Verification items for the finished model (mm, model axes). A direction names the side the tool comes from. Give positions to 0.01 mm unless a question says otherwise; leave off trailing zeros. Write each loop counter-clockwise with the first axis right and the second up, starting at its lowest first coordinate (ties: lowest second). Pieces come first, ordered by that corner, then holes.
from build123d import *

# Parameters (mm, degrees)
F0_R     = 1.55
F1_DEPTH = 2.5
F3_DEPTH = 2.501
F4_W     = 6.5
F4_H     = 1
F5_DEPTH = 1
F6_W     = 6.5
F6_H     = 1
F7_DEPTH = 1
F8_SIZE  = 0.99999


# Not quite as in the source:
# - a fillet or chamfer is up to 0.001 mm smaller than in the source, because OpenCascade refuses the exact size


with BuildPart() as f1:
    # F0 (on Top) → F1 (new body)
    with BuildSketch(Plane.XY):
        with BuildLine():
            Line((7, 4), (-7, 4))
            ThreePointArc((-7, 4), (-9.8284271247, 2.8284271247), (-11, 0))
            ThreePointArc((-11, 0), (-9.8284271247, -2.8284271247), (-7, -4))
            Line((-7, -4), (7, -4))
            ThreePointArc((7, -4), (9.8284271247, -2.8284271247), (11, 0))
            ThreePointArc((11, 0), (9.8284271247, 2.8284271247), (7, 4))
        make_face()
        with Locations((-7, 0)):
            Circle(F0_R, mode=Mode.SUBTRACT)
        with Locations((7, 0)):
            Circle(F0_R, mode=Mode.SUBTRACT)
    extrude(amount=F1_DEPTH)

    # F2 (on face) → F3 (cut, through all)
    with BuildSketch(Plane.XY.offset(2.5)):
        with BuildLine():
            Line((-7, 1.55), (-7, 4))
            ThreePointArc((-7, 4), (-11, 0), (-7, -4))
            Line((-7, -4), (-7, -1.55))
            ThreePointArc((-7, -1.55), (-8.55, 0), (-7, 1.55))
        make_face()
        with BuildLine():
            ThreePointArc((7, -4), (11, 0), (7, 4))
            Line((7, 4), (7, 1.55))
            ThreePointArc((7, 1.55), (8.0960155108, 1.0960155108), (8.55, 0))
            ThreePointArc((8.55, 0), (8.0960155108, -1.0960155108), (7, -1.55))
            Line((7, -1.55), (7, -4))
        make_face()
    extrude(amount=-F3_DEPTH, mode=Mode.SUBTRACT)

    # F4 (on face) → F5 (cut)
    with BuildSketch(Plane.XY.offset(2.5)):
        with Locations((0, 1.5)):
            Rectangle(F4_W, F4_H)
        with Locations((0, -2.5)):
            Rectangle(F4_W, F4_H)
        with Locations((0, -0.5)):
            Rectangle(F4_W, F4_H)
        with Locations((0, 3.5)):
            Rectangle(F4_W, F4_H)
    extrude(amount=-F5_DEPTH, mode=Mode.SUBTRACT)

    # F6 (on face) → F7 (cut)
    with BuildSketch(Plane(origin=(0, 0, 0), x_dir=(1, 0, 0), z_dir=(0, 0, -1))):
        with Locations((0, -0.5)):
            Rectangle(F6_W, F6_H)
        with Locations((0, 3.5)):
            Rectangle(F6_W, F6_H)
        with Locations((0, 1.5)):
            Rectangle(F6_W, F6_H)
        with Locations((0, -2.5)):
            Rectangle(F6_W, F6_H)
    extrude(amount=-F7_DEPTH, mode=Mode.SUBTRACT)

    # F8 (size 1 in the source; OpenCascade refuses exactly that, so slightly less here)
    f8_edges = [f1.edges().sort_by_distance(p)[0] for p in [
        (0, 3, 0),
        (0, 1, 0),
        (0, -1, 0),
        (0, -3, 0),
        (0, -4, 2.5),
        (0, -2, 2.5),
        (0, 0, 2.5),
        (0, 2, 2.5),
    ]]
    chamfer(f8_edges, length=F8_SIZE)


solid = f1.part
Item 1: Sectioned sample at B-B on z = 1.2. Record the cut outline in (x, y), then the cut area to 3 significant figures.
Answer key:
outline: (-7, -4) - (7, -4) - (7, -1.55) arc R1.55 cw to (7, 1.55) - (7, 4) - (-7, 4) - (-7, 1.55) arc R1.55 cw to (-7, -1.55) - close
area: 104 mm2
Item 2: Depth check by flat-ended pin: pin 1 (1.1 mm diameter, centred on x = -0.5, z = 2, fed in from +Y); pin 2 (1.1 mm diameter, centred on y = 0, z = 2, fed in from +X). Enter the tip coordinate at first touch or a pass-through.
Answer key:
pin 1: stops at y = 4
pin 2: stops at x = 5.55
Item 3: Sectioned sample at A-A on y = 2.5. Record the cut outline in (x, z), then the cut area to 4 significant figures.
Answer key:
outline: (-7, 0) - (-3.25, 0) - (-3.25, 1) - (3.25, 1) - (3.25, 0) - (7, 0) - (7, 2.5) - (3.25, 2.5) - (3.25, 2) - (-3.25, 2) - (-3.25, 2.5) - (-7, 2.5) - close
area: 25.25 mm2
Item 4: Release check for a two-part mould opening along Y. For faces 1 (the face through (-0.1, -4, 1.2)), 2 (the face through (-7, -3, 1)), 3 (the face through (0, -0.5, 1.5)) record: released by +Y, released by -Y, zero draft, split by the parting line, or undercut.
Answer key:
face 1: released by -Y
face 2: zero draft
face 3: undercut
Item 5: Sectioned sample at D-D on y = -2.75. Record the cut outline in (x, z).
Answer key:
outline: (-7, 0) - (-3.25, 0) - (-3.25, 0.75) - (3.25, 0.75) - (3.25, 0) - (7, 0) - (7, 2.5) - (3.25, 2.5) - (3.25, 1.5) - (-3.25, 1.5) - (-3.25, 2.5) - (-7, 2.5) - close
Item 6: Scan lines: line 1 along Y through (x, z) = (-1.25, 1.9); line 2 along X through (y, z) = (-2, 1.6); line 3 along Y through (x, z) = (-1, 1.65). Record each from-to range of solid material in increasing order.
Answer key:
line 1: y = -3.6 to -3, -1.6 to -1, 0.4 to 1, 2.4 to 3
line 2: x = -7 to -3.25, 3.25 to 7
line 3: y = -3.85 to -3, -1.85 to -1, 0.15 to 1, 2.15 to 3
Item 7: Sectioned sample at C-C on z = 2.15. Record the cut outline in (x, y).
Answer key:
outline: (-7, -3.35) - (7, -3.35) - (7, -1.55) arc R1.55 cw to (7, 1.55) - (7, 4) - (3.25, 4) - (3.25, 3) - (-3.25, 3) - (-3.25, 4) - (-7, 4) - (-7, 1.55) arc R1.55 cw to (-7, -1.55) - close; hole (-3.25, -3) - (3.25, -3) - (3.25, -1.35) - (-3.25, -1.35) - close; hole (-3.25, -1) - (3.25, -1) - (3.25, 0.65) - (-3.25, 0.65) - close; hole (-3.25, 1) - (3.25, 1) - (3.25, 2.65) - (-3.25, 2.65) - close
Item 8: Set-up check for faces 4 (the face through (0, -1.5, 1)), 5 (the face through (-3.25, -3.2, 0.5)), 6 (the face through (0, 2.5, 2)), 7 (the face through (7, 3, 1)), 8 (the face through (5.45, 0.03, 1.23)): record each of +Z, -Z, +X, -X, +Y, -Y from which the full face is reachable in a straight line by a thin tool's end or side.
Answer key:
face 4: -Z
face 5: -Z, -Y
face 6: +Z
face 7: +Z, -Z, +X, +Y, -Y
face 8: +Z, -Z, +X
